Model file for the job. Use its own axes, mm. Face numbers are marked on the shaded views. A direction names the side the tool comes from. Coordinates: 2 decimals unless noted, no trailing zeros. Write each loop counter-clockwise with the first axis right and the second up, starting at its lowest first coordinate (ties: lowest second). Pieces come first, ordered by that corner, then holes. Notation, with made-up numbers: (-37.75, 80) -> (-13.75, 80) arc R28 cw to (-13.75, 117) -> close; hole circle Ø10 at (-23.5, -5). An arc over 180 degrees is marked (long way). Answer as a JSON object with one key per item and string values. Group by question number.
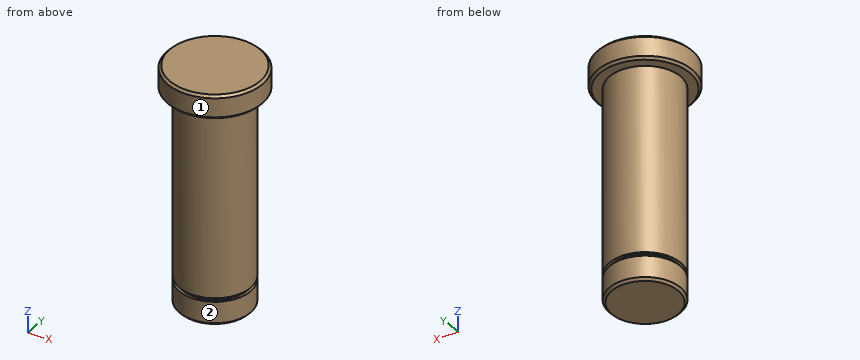
from build123d import *

# Parameters (mm, degrees)
SKETCH_1_R      = 15
EXTRUDE_1_DEPTH = 90
SKETCH_2_R      = 20
EXTRUDE_2_DEPTH = 10
SKETCH_3_W      = 4.032113995
SKETCH_3_H      = 1.5
CHAMFER_1_SIZE  = 1


with BuildPart() as part:
    # 草图1 → 凸台-拉伸1 (new body)
    with BuildSketch(Plane.XY):
        with Locations(Location((0, 0, 0), (0, 0, 180))):
            Circle(SKETCH_1_R)
    extrude(amount=EXTRUDE_1_DEPTH)

    # 草图2 → 凸台-拉伸2 (add)
    with BuildSketch(Plane.XY.offset(90)):
        Circle(SKETCH_2_R)
    extrude(amount=EXTRUDE_2_DEPTH)

    # 草图3 → 切除-旋转1 (revolve, cut)
    with BuildSketch(Plane(origin=(0, 0, 0), x_dir=(1, 0, 0), z_dir=(0, 1, 0))):
        with Locations((-15.816056998, -10.75)):
            Rectangle(SKETCH_3_W, SKETCH_3_H)
    revolve(axis=Axis((0, 0, 0), (0, 0, 1)), mode=Mode.SUBTRACT)

    # 倒角1
    chamfer_1_edges = [part.edges().sort_by_distance(p)[0] for p in [
        (15, 0, 0),
        (-20, 0, 90),
        (-20, 0, 100),
    ]]
    chamfer(chamfer_1_edges, length=CHAMFER_1_SIZE)


solid = part.part
(1) Wall check: probe 1 along Y at (x, z) = (0, 7.5); probe 2 along Z at (x, y) = (16, -5.5); probe 3 along X at (y, z) = (12, 63). Give the ranges that are in metal, low to high.
(2) 3-axis set-ups, long thin cutter, end or side, ignore diameter. For the marked faces 1 and 2: which of +Z, -Z, +X, -X, +Y, -Y reach the whole face in a straight line?
(3) Pin check, flat tips, straight feed: pin 1 (1.5 mm diameter, centred on y = -11, z = 83.5, fed in from +X); pin 2 (1 mm diameter, centred on x = 8, z = 52, fed in from +Y); pin 3 (12 mm diameter, centred on x = -4, z = 33, fed in from +Y). Stop position of each tip, or through.
(4) Cut at C-C on z = 88.5. List the corners of the cut face in (x, y).
(5) Cut at A-A on x = 0. List the corners of the cut face in (y, z), plus the area to 3 significant figures.
Results found:
{
 "1": {"probe 1": "y = -15 to 15", "probe 2": "z = 90 to 100", "probe 3": "x = -9 to 9"},
 "2": {"face 1": "+Z, -Z", "face 2": "-Z"},
 "3": {"pin 1": "stops at x = 10.95", "pin 2": "stops at y = 12.99", "pin 3": "stops at y = 15"},
 "4": {"outline": "circle Ø30 at (0, 0)"},
 "5": {"outline": "(-20, 91) -> (-19, 90) -> (-15, 90) -> (-15, 11.5) -> (-13.8, 11.5) -> (-13.8, 10) -> (-15, 10) -> (-15, 1) -> (-14, 0) -> (14, 0) -> (15, 1) -> (15, 10) -> (13.8, 10) -> (13.8, 11.5) -> (15, 11.5) -> (15, 90) -> (19, 90) -> (20, 91) -> (20, 99) -> (19, 100) -> (-19, 100) -> (-20, 99) -> close", "area": "3,090 mm²"}
}
